```python
from build123d import *

# Parameters (mm, degrees)
F0_W     = 65
F0_H     = 45
F0_R     = 3.25
F1_DEPTH = 12
F2_SIZE  = 0.5


with BuildPart() as f1:
    # F0 (on Front) → F1 (new body)
    with BuildSketch(Plane.XZ):
        Rectangle(F0_W, F0_H)
        with Locations((-24, -14)):
            Circle(F0_R, mode=Mode.SUBTRACT)
        with Locations((-12, -14)):
            Circle(F0_R, mode=Mode.SUBTRACT)
        with Locations((12, -14)):
            Circle(F0_R, mode=Mode.SUBTRACT)
        with Locations((24, -14)):
            Circle(F0_R, mode=Mode.SUBTRACT)
        with Locations((-24, 14)):
            Circle(F0_R, mode=Mode.SUBTRACT)
        with Locations((-12, 14)):
            Circle(F0_R, mode=Mode.SUBTRACT)
        with Locations((12, 14)):
            Circle(F0_R, mode=Mode.SUBTRACT)
        with Locations((24, 14)):
            Circle(F0_R, mode=Mode.SUBTRACT)
    extrude(amount=F1_DEPTH)

    # F2
    f2_edges = [f1.edges().sort_by_distance(p)[0] for p in [
        (-20.75, -6, 14),
        (-27.25, 0, 14),
        (-27.25, -12, 14),
        (-8.75, -6, 14),
        (-15.25, 0, 14),
        (-15.25, -12, 14),
        (-20.75, -6, -14),
        (-27.25, 0, -14),
        (-27.25, -12, -14),
        (-8.75, -6, -14),
        (-15.25, 0, -14),
        (-15.25, -12, -14),
        (15.25, -6, 14),
        (8.75, 0, 14),
        (8.75, -12, 14),
        (27.25, -6, 14),
        (20.75, 0, 14),
        (20.75, -12, 14),
        (27.25, -6, -14),
        (20.75, 0, -14),
        (20.75, -12, -14),
        (15.25, -6, -14),
        (8.75, 0, -14),
        (8.75, -12, -14),
    ]]
    chamfer(f2_edges, length=F2_SIZE)


solid = f1.part
```
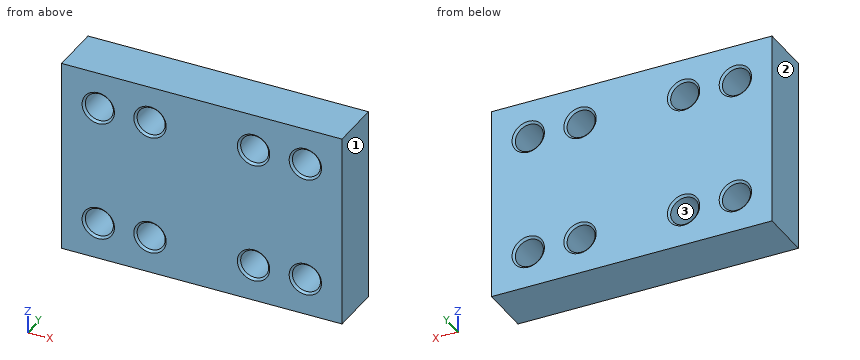
Can you work these out from the model? Positions are in its coordinate system, mm. Face numbers are marked on the shaded views. Round coordinates to 2 decimals unless told otherwise and drop trailing zeros. Loops run counter-clockwise (first coordinate to the right, second up) from the corner with the lowest first, then second, coordinate; pieces in that order, holes last. Notation, with made-up numbers: M 48.25,-19.75 L 65.25,-19.75 A21 ccw 65.25,17.25 Z; hole C 77,25 d3. An arc over 180 degrees is marked long. Answer as a JSON object with one key per item and string values. Group by question number.
Q1. Imagine slicing it at B-B, the plane y = -1.5. Count the separate pieces of the cut face and the enclosed holes in it, then the cut area to 3 significant figures.
Q2. Imagine slicing it at A-A, the plane x = -24. Please give me the cut outline in (y, z), then the cut area to 3 significant figures.
Q3. Please list where these lines run through material, in increasing order: L1, parallel to Z at x = -12, y = -8.25; L2, parallel to Z at x = 15, y = -9; L3, parallel to Y at x = -27, z = -12.5.
Q4. Will this pin go through, and if not, where does the flat tip stop? pin 1 (2 mm diameter, centred on x = -9.5, z = -16, fed in from +Y).
Q5. We'd pull the mould along X, two halves only. Please class the marked faces 1, 2 and 3: +X half, -X half, draft (parallel to the pull), parting line (faces both ways), or undercut.
Findings:
{
 "1": {"separate pieces": "1", "enclosed holes": "8", "area": "2,660 mm2"},
 "2": {"outline": "M -12,-22.5 L 0,-22.5 L 0,-17.75 L -0.5,-17.25 L -11.5,-17.25 L -12,-17.75 Z; M -12,-10.25 L -11.5,-10.75 L -0.5,-10.75 L 0,-10.25 L 0,10.25 L -0.5,10.75 L -11.5,10.75 L -12,10.25 Z; M -12,17.75 L -11.5,17.25 L -0.5,17.25 L 0,17.75 L 0,22.5 L -12,22.5 Z", "area": "383 mm2"},
 "3": {"L1": "z = -22.5 to -17.25, -10.75 to 10.75, 17.25 to 22.5", "L2": "z = -22.5 to -15.25, -12.75 to 12.75, 15.25 to 22.5", "L3": "y = -11.6 to -0.4"},
 "4": {"pin 1": "stops at y = 0"},
 "5": {"face 1": "+X half", "face 2": "-X half", "face 3": "undercut"}
}
